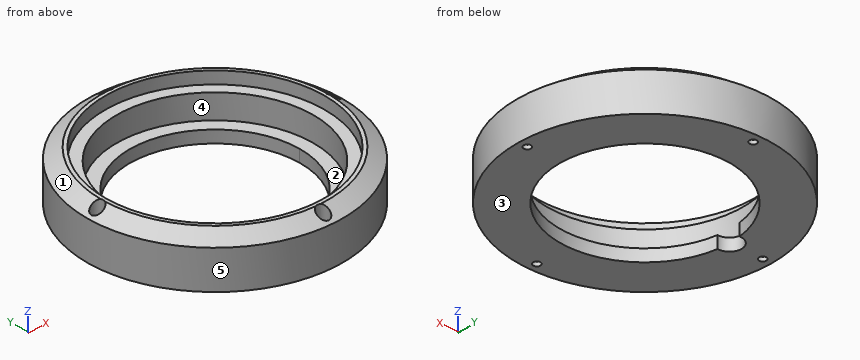
```python
from build123d import *

# Parameters (mm, degrees)
F0_R           = 52.5
F0_R_2         = 35
F1_DEPTH       = 20
F2_DEPTH       = 20
F3_R           = 45.0292723638
F3_R_2         = 35
F4_DEPTH       = 5
F5_SIZE2       = 4.2012452293
F5_SIZE        = 6
F7_D           = 3
F7_START       = 3.3259859
F7_CBORE_D     = 5
F7_CBORE_DEPTH = 15
F8_R           = 40.3913127828
F9_DEPTH       = 10
F10_DEPTH      = 50


with BuildPart() as f1:
    # F0 (on Top) → F1 (new body)
    with BuildSketch(Plane.XY):
        Circle(F0_R)
        Circle(F0_R_2, mode=Mode.SUBTRACT)
        Circle(F0_R_2)
    extrude(amount=F1_DEPTH)

    # F0 (on Top) → F2 (cut)
    with BuildSketch(Plane.XY):
        Circle(F0_R_2)
    extrude(amount=F2_DEPTH, mode=Mode.SUBTRACT)

    # F3 (on face) → F4 (cut)
    with BuildSketch(Plane.XY.offset(20)):
        Circle(F3_R)
        Circle(F3_R_2, mode=Mode.SUBTRACT)
    extrude(amount=-F4_DEPTH, mode=Mode.SUBTRACT)

    # F5
    f5_edges = [f1.edges().sort_by_distance(p)[0] for p in [
        (-52.5, 0, 20),
    ]]
    f5_side = f1.faces().sort_by_distance((-51.015076, 0, 20))[0]
    chamfer(f5_edges, length=F5_SIZE, length2=F5_SIZE2, reference=f5_side)

    # F7 (through all)
    # its depths count from where the whole tool has entered the part; down to there all is cleared
    with Locations(Plane.XY.offset(20).offset(-F7_START)):
        with Locations((-48.75, 0), (0, -48.75), (48.75, 0), (0, 48.75)):
            CounterBoreHole(F7_D / 2, F7_CBORE_D / 2, F7_CBORE_DEPTH)

    # F8 (on face) → F9 (cut)
    with BuildSketch(Plane.XY.offset(15)):
        Circle(F8_R)
        with BuildLine():
            ThreePointArc((-34.6428571429, -4.9872285871), (-40, 0), (-34.6428571429, 4.9872285871))
            ThreePointArc((-34.6428571429, 4.9872285871), (2.5, 34.9106001094), (35, 0))
            ThreePointArc((35, 0), (2.5, -34.9106001094), (-34.6428571429, -4.9872285871))
        make_face(mode=Mode.SUBTRACT)
    extrude(amount=-F9_DEPTH, mode=Mode.SUBTRACT)

    # F10 (cut): a face of the model
    f10_faces = [f1.faces().sort_by_distance(p)[0] for p in [
        (-37.0564415312, 0, 15),
    ]]
    extrude(f10_faces, amount=-F10_DEPTH, mode=Mode.SUBTRACT)


solid = f1.part
```
Could you check a few things on this model? Use its own coordinates, in mm. Face numbers are marked on the shaded views. A direction names the side the tool comes from. Coordinates: 2 decimals unless noted, no trailing zeros. Order: outer loops, then holes, each group sorted by start corner. A loop starts at its lowest first (then second) coordinate and runs counter-clockwise, first axis right, second up. Notation, with made-up numbers: M 48.25,33 L 73.25,33 A22 cw 73.25,48 Z; hole C -23,-19.5 d2. An arc over 180 degrees is marked long. Use a Markdown table: item, result. Add a question column.
Q1. We'd pull the mould along X, two halves only. Please class the marked faces 1, 2 and 3: pulls with the +X half, pulls with the -X half, needs draft (parallel to the pull), parting line crosses it, or undercut.
Q2. Which directions (+Z, -Z, +X, -X, +Y, -Y) give clear straight access to the entire face, cutting with the end or side of a thin tool? Please do the marked faces 4 and 5.
Q3. If I drill on L1, parallel to Y at x = 0, z = 1.15; L2, parallel to Y at x = 0, z = 13.25; L3, parallel to Z at x = -28.5, y = 23.5, over which ranges is the centre line in solid material (lowest first)?
Q4. I want a section at A-A on z = 13.75. List the corners of the cut face in (x, y) for me.
Q5. I'm going to push flat-ended pins straight in: pin 1 (10 mm diameter, centred on y = 10.5, z = 5.5, fed in from -X); pin 2 (8 mm diameter, centred on y = 38, z = 2.5, fed in from -X); pin 3 (6.5 mm diameter, centred on x = 48.75, y = 0, fed in from -Z); pin 4 (2.5 mm diameter, centred on x = 48, y = 0, fed in from +Z). Where does each tip first touch, or does it pass through?
Checked values:
| question | item | result |
|---|---|---|
| 1 | face 1 | parting line crosses it |
| 1 | face 2 | undercut |
| 1 | face 3 | needs draft |
| 2 | face 4 | +Z |
| 2 | face 5 | +Z, -Z |
| 3 | L1 | -52.5 to -50.25, -47.25 to -35, 35 to 47.25, 50.25 to 52.5 |
| 3 | L2 | -52.5 to -51.25, -46.25 to -40.39, 40.39 to 46.25, 51.25 to 52.5 |
| 3 | L3 | 0 to 5 |
| 4 | outline | C 0,0 d105; hole C -48.75,0 d5; hole C 0,0 d80.78; hole C 0,-48.75 d5; hole C 0,48.75 d5; hole C 48.75,0 d5 |
| 5 | pin 1 | x = -52.21 |
| 5 | pin 2 | x = -40 |
| 5 | pin 3 | z = 0 |
| 5 | pin 4 | z = 1.67 |
